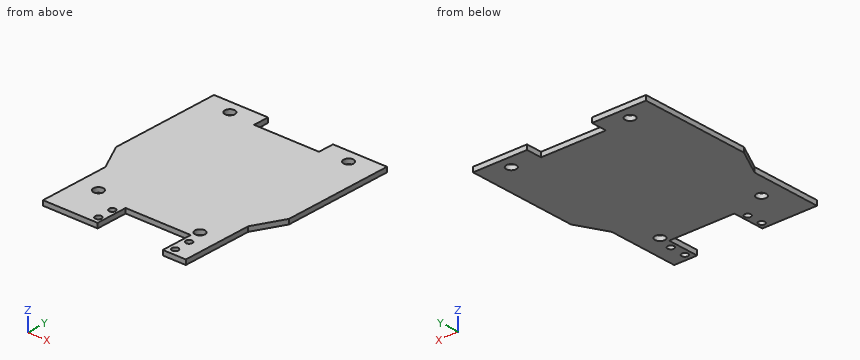
```python
from build123d import *

# Parameters (mm, degrees)
SKETCH1_R           = 3.125
BOSS_EXTRUDE1_DEPTH = 3
SKETCH2_R           = 2
CUT_EXTRUDE1_DEPTH  = 3
SKETCH3_R           = 3.125
CUT_EXTRUDE2_DEPTH  = 3


with BuildPart() as part:
    # Sketch1 → Boss-Extrude1 (new body)
    with BuildSketch(Plane.XY):
        Polygon((-17.171078522, 8.102088167), (16.942973826, 8.102088167), (16.942973826, -1.897911833), (57.945, -1.897911833), (57.945, 8.102088167), (92.055, 8.102088167), (92.055, -61.897911833), (82.525114176, -80.288734737), (82.525114176, -124.897911833), (68.025114176, -124.897911833), (68.025114176, -104.897911833), (26.858807303, -104.897911833), (26.858807303, -124.897911833), (-7.641192697, -124.897911833), (-7.641192697, -80.288734737), (-17.171078522, -61.897911833), align=None)
        Circle(SKETCH1_R, mode=Mode.SUBTRACT)
        with Locations((75, 0)):
            Circle(SKETCH1_R, mode=Mode.SUBTRACT)
    extrude(amount=BOSS_EXTRUDE1_DEPTH)

    # Sketch2 → Cut-Extrude1 (cut)
    with BuildSketch(Plane.XY.offset(3)):
        with Locations((71.951514176, -120.540427833)):
            Circle(SKETCH2_R)
        with Locations((71.951514176, -110.541227833)):
            Circle(SKETCH2_R)
        with Locations((23.455105176, -120.540427833)):
            Circle(SKETCH2_R)
        with Locations((23.455105176, -110.541227833)):
            Circle(SKETCH2_R)
    extrude(amount=-CUT_EXTRUDE1_DEPTH, mode=Mode.SUBTRACT)

    # Sketch3 → Cut-Extrude2 (cut)
    with BuildSketch(Plane(origin=(0, 0, 0), x_dir=(-1, 0, 0), z_dir=(0, 0, -1))):
        with Locations((-69.500000176, -100.000011833)):
            Circle(SKETCH3_R)
        with Locations((-5.387973651, -100.000011833)):
            Circle(SKETCH3_R)
    extrude(amount=-CUT_EXTRUDE2_DEPTH, mode=Mode.SUBTRACT)


solid = part.part
```
Here's how the part is built. I have some questions about the finished solid (model axes, mm). Coordinates: 2 decimals unless noted, no trailing zeros. Order: outer loops, then holes, each group sorted by start corner. A loop starts at its lowest first (then second) coordinate and runs counter-clockwise, first axis right, second up.
1) Imagine slicing it at A-A on x = 0. List the corners of the cut face in (y, z) for me (3 decimals), and give its area (3 significant figures).
2) Will these pins go through, and if not, where does the flat tip stop? pin 1 (0.9 mm diameter, centred on x = 43.5, z = 2, fed in from +Y); pin 2 (0.9 mm diameter, centred on y = -113, z = 2, fed in from +X); pin 3 (0.9 mm diameter, centred on x = 51.5, z = 1, fed in from -Y).
3) Imagine slicing it at C-C on z = 1.6. State how many separate pieces and enclosed holes the cut face has, and give its area (3 significant figures).
4) Imagine slicing it at B-B on y = 0. List the corners of the cut face in (x, z) for me (3 decimals), and give its area (3 significant figures).
5) Imagine slicing it at D-D on x = 55.5. List the corners of the cut face in (y, z) for me.
6) I need wall thicknesses on line 1 (X direction, y = -113, z = 1.3); line 2 (Y direction, x = 0, z = 1) (3 decimals); line 3 (Y direction, x = 32, z = 2.55). Which ranges of each line are inside material? Lowest first, please.
Response values:
1. outline: (-124.898, 0) - (-3.125, 0) - (-3.125, 3) - (-124.898, 3) - close; (3.125, 0) - (8.102, 0) - (8.102, 3) - (3.125, 3) - close
1. area: 380 mm2
2. pin 1: stops at y = -1.9
2. pin 2: stops at x = 82.53
2. pin 3: stops at y = -104.9
3. separate pieces: 1
3. enclosed holes: 8
3. area: 12,100 mm2
4. outline: (-17.171, 0) - (-3.125, 0) - (-3.125, 3) - (-17.171, 3) - close; (3.125, 0) - (16.943, 0) - (16.943, 3) - (3.125, 3) - close; (57.945, 0) - (71.875, 0) - (71.875, 3) - (57.945, 3) - close; (78.125, 0) - (92.055, 0) - (92.055, 3) - (78.125, 3) - close
4. area: 167 mm2
5. outline: (-104.9, 0) - (-1.9, 0) - (-1.9, 3) - (-104.9, 3) - close
6. line 1: x = -7.64 to 26.86, 68.03 to 82.53
6. line 2: y = -124.898 to -3.125, 3.125 to 8.102
6. line 3: y = -104.9 to -1.9
